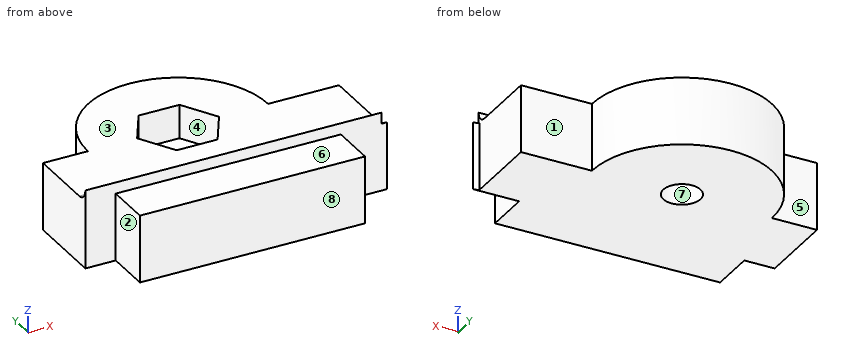
from build123d import *

# Parameters (mm, degrees)
BOSS_EXTRUDE1_DEPTH = 6
BOSS_EXTRUDE2_DEPTH = 26.3
BOSS_EXTRUDE3_DEPTH = 6
SKETCH8_R           = 1.65
BOSS_EXTRUDE4_DEPTH = 3


with BuildPart() as part:
    # Sketch1 → Boss-Extrude1 (new body)
    with BuildSketch(Plane.XY):
        with BuildLine():
            Line((0, 0), (20, 0))
            Line((20, 0), (20, 4))
            Line((20, 4), (23.6, 4))
            Line((23.6, 4), (23.6, 11))
            Line((23.6, 11), (17.3, 11))
            ThreePointArc((17.3, 11), (9.3, 19), (1.3, 11))
            Line((1.3, 11), (-2.7, 11))
            Line((-2.7, 11), (-2.7, 4))
            Line((-2.7, 4), (0, 4))
            Line((0, 4), (0, 0))
        make_face()
        Polygon((11.118653348, 14.15), (7.481346652, 14.15), (5.662693304, 11), (7.481346652, 7.85), (11.118653348, 7.85), (12.937306696, 11), align=None, mode=Mode.SUBTRACT)
    extrude(amount=BOSS_EXTRUDE1_DEPTH)

    # Sketch2 → Boss-Extrude2 (add)
    with BuildSketch(Plane.ZY.offset(2.7)):
        with BuildLine():
            Line((6, 4), (6, 5))
            ThreePointArc((6, 5), (6.292893219, 4.292893219), (7, 4))
            Line((7, 4), (6, 4))
        make_face()
    extrude(amount=-BOSS_EXTRUDE2_DEPTH)

    # Sketch4 → Boss-Extrude3 (add)
    with BuildSketch(Plane.XY.offset(6)):
        with BuildLine():
            Line((23.1, 4), (23.1, 5))
            ThreePointArc((23.1, 5), (23.392893219, 4.292893219), (24.1, 4))
            Line((24.1, 4), (23.1, 4))
        make_face()
        with BuildLine():
            Line((-1.5, 4), (-2.5, 4))
            ThreePointArc((-2.5, 4), (-1.792893219, 4.292893219), (-1.5, 5))
            Line((-1.5, 5), (-1.5, 4))
        make_face()
    extrude(amount=-BOSS_EXTRUDE3_DEPTH)

    # Sketch8 → Boss-Extrude4 (add)
    with BuildSketch(Plane.XY):
        Polygon((7.481346652, 14.15), (5.662693304, 11), (7.481346652, 7.85), (11.118653348, 7.85), (12.937306696, 11), (11.118653348, 14.15), align=None)
        with Locations((9.3, 11)):
            Circle(SKETCH8_R, mode=Mode.SUBTRACT)
    extrude(amount=BOSS_EXTRUDE4_DEPTH)


solid = part.part
Build history of the part. All positions in model axes, mm. Face numbers are marked on the shaded views. A direction names the side the tool comes from. Coordinates: 2 decimals unless noted, no trailing zeros. Order: outer loops, then holes, each group sorted by start corner. A loop starts at its lowest first (then second) coordinate and runs counter-clockwise, first axis right, second up. Notation, with made-up numbers: (18.5, 83.25) - (44.5, 83.25) arc R19 cw to (44.5, 102.25) - close; hole circle Ø1 at (-4.5, 80). An arc over 180 degrees is marked (long way). Put each result on its own line as item: value.
1. Saw through at C-C (x = 18). Write the cut outline in (y, z), and give its area (3 significant figures).
Answer sheet:
outline: (0, 0) - (11, 0) - (11, 6) - (5, 6) arc R1 cw to (4, 7) - (4, 6) - (0, 6) - close
area: 66.2 mm^2
2. Saw through at D-D (z = 1.75). Write the cut outline in (x, y).
Answer sheet:
outline: (-2.7, 4) - (0, 4) - (0, 0) - (20, 0) - (20, 4) - (24.1, 4) arc R1 cw to (23.6, 4.13) - (23.6, 11) - (17.3, 11) arc R8 ccw to (1.3, 11) - (-2.7, 11) - close; hole circle Ø3.3 at (9.3, 11)
3. Probe line 1 along Y through (x, z) = (9.3, 0.75); line 2 along Y through (x, z) = (9, 5.5); line 3 along Z through (x, y) = (10.5, 6). List the from-to ranges inside material, lowest first. Write a range as [from, to].
Answer sheet:
line 1: y = [0, 9.35], [12.65, 19]
line 2: y = [0, 7.85], [14.15, 18.99]
line 3: z = [0, 6]
4. Saw through at A-A (x = 9.3). Write the cut outline in (y, z).
Answer sheet:
outline: (0, 0) - (9.35, 0) - (9.35, 3) - (7.85, 3) - (7.85, 6) - (5, 6) arc R1 cw to (4, 7) - (4, 6) - (0, 6) - close; (12.65, 0) - (19, 0) - (19, 6) - (14.15, 6) - (14.15, 3) - (12.65, 3) - close
5. Pull direction Y, two halves, no side cores. Call the marked faces 5, 6, 7 and 8: pulls with the +Y half, pulls with the -Y half, needs draft (parallel to the pull), parting line crosses it, or undercut.
Answer sheet:
face 5: pulls with the +Y half
face 6: needs draft
face 7: undercut
face 8: pulls with the -Y half
6. Tool access for the marked faces 1, 2, 3 and 4: list every direction of +Z, -Z, +X, -X, +Y, -Y with a clear straight run to the whole face (end or side of a thin tool).
Answer sheet:
face 1: +Z, -Z, +X, +Y
face 2: +Z, -Z, -X, -Y
face 3: +Z, +X, -X, +Y
face 4: +Z
7. Saw through at B-B (z = 4.5). Write the cut outline in (x, y).
Answer sheet:
outline: (-2.7, 4) - (0, 4) - (0, 0) - (20, 0) - (20, 4) - (24.1, 4) arc R1 cw to (23.6, 4.13) - (23.6, 11) - (17.3, 11) arc R8 ccw to (1.3, 11) - (-2.7, 11) - close; hole (5.66, 11) - (7.48, 7.85) - (11.12, 7.85) - (12.94, 11) - (11.12, 14.15) - (7.48, 14.15) - close
8. Drop flat-ended pins along their axis: P1, Ø4.5, axis at x = 6, y = 1.5, coming from the +Z side; P2, Ø1.2, axis at y = 3, z = 4, coming from the -X side; P3, Ø4, axis at x = 0.5, z = 3, coming from the +Y side. Give the stop position or say it passes through.
Answer sheet:
P1: stops at z = 6
P2: stops at x = 0
P3: stops at y = 15.21
